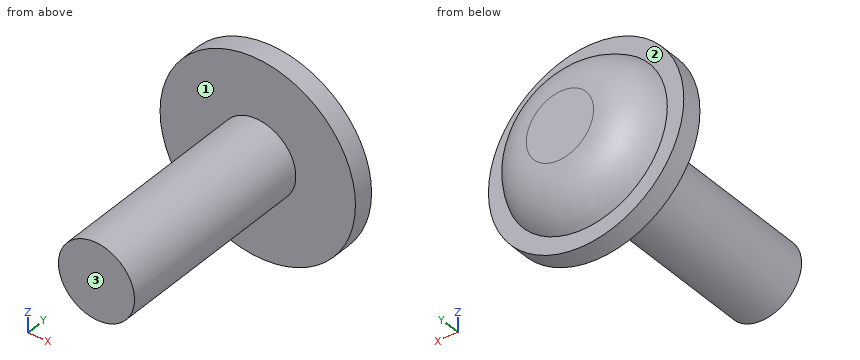
Autodesk Inventor part; units mm, degrees
ref_plane "YZ Plane" through (0, 0, 0) normal (1, 0, 0) x (0, 1, 0)
ref_plane "XZ Plane" through (0, 0, 0) normal (0, 1, 0) x (-1, 0, 0)
ref_plane "XY Plane" through (0, 0, 0) normal (0, 0, 1) x (1, 0, 0)
sketch "スケッチ1" plane through (0, 0, 0) normal (0, 1, 0) x (-1, 0, 0)
  circle A0 centre (0, 0) radius 3.85
  circle A1 centre (0, 0) radius 1.5
  circle A2 centre (0, 0) radius 3.2
  dimension "d0" = 7.7
  dimension "d1" = 3
  dimension "d6" = 6.4
extrude "押し出し1" add sketch "スケッチ1" against normal blind 8 contours A1
extrude "押し出し2" add sketch "スケッチ1" along normal blind 0.8 contours A0 | A1 | A2
extrude "押し出し3" add sketch "スケッチ1" along normal blind 2.1 contours A1 | A2
fillet "フィレット1" radius 2 1 edges at (3.2, 2.1, 0)
thread "ねじ1"
properties part number "ClampHorn_Screw"
Geometry check sheet. Reference: the model listing, model coordinates, mm. Face numbers are marked on the shaded views. A direction names the side the tool comes from. Give positions to 0.01 mm unless a question says otherwise; leave off trailing zeros. Order: outer loops, then holes, each group sorted by start corner. A loop starts at its lowest first (then second) coordinate and runs counter-clockwise, first axis right, second up.
1. Thickness scan on L1, parallel to Y at x = -1.75, z = 3.25; L2, parallel to X at y = 1, z = 1.5; L3, parallel to Z at x = 0.5, y = -0.5. Record the ranges inside material, lowest first.
2. Section check A-A, the plane y = -5.5. Enter the section's corners in (x, z), and give its area (3 significant figures).
3. Access from +Z, -Z, +X, -X, +Y, -Y to the whole of each face (thin tool, end or side, straight path). Record for the marked faces 1, 2 and 3.
4. Gauge pin test, flat ends, axial feed: pin 1 Ø3 at (x, z) = (2.5, -2) entering from -Y; pin 2 Ø1.5 at (x, z) = (-2, -3) entering from +Y; pin 3 Ø3 at (x, y) = (1.5, -1) entering from +Z. Record the tip position at first contact, or that the pin passes through.
Values follow:
1. L1: y = 0 to 0.8
1. L2: x = -2.73 to 2.73
1. L3: z = -1.41 to 1.41
2. outline: circle Ø3 at (0, 0)
2. area: 7.07 mm2
3. face 1: -Y
3. face 2: +Y
3. face 3: +Z, -Z, +X, -X, -Y
4. pin 1: stops at y = 0
4. pin 2: stops at y = 1.39
4. pin 3: stops at z = 3.83
